The model under review builds one solid part; all positions refer to its coordinate system, in mm. A direction names the side the tool comes from. Coordinates: 2 decimals unless noted, no trailing zeros. Write each loop counter-clockwise with the first axis right and the second up, starting at its lowest first coordinate (ties: lowest second). Pieces come first, ordered by that corner, then holes. Notation, with made-up numbers: M 19.5,-17.75 L 28.5,-17.75 A37 cw 28.5,19.25 Z; hole C 58,70 d3. An arc over 180 degrees is marked long. Answer as a JSON object with one key per item and string values.
```python
from build123d import *
from build123d import SkipClean  # not in build123d's __all__

# Parameters (mm, degrees)
F1_DEPTH  = 24.13
F2_R      = 2.032
F2_R_2    = 1.2065
F3_DEPTH  = 0.7874
F4_DEPTH  = 25.4
F6_DEPTH  = 0.5
F7_DEPTH  = 2
F8_DEPTH  = 2
F9_W      = 25.654
F9_H      = 1
F10_DEPTH = 1.27
F11_R     = 1.2065
F12_DEPTH = 1.905
F13_DEPTH = 1.905
F14_DEPTH = 1.0414


# Not quite as in the source:
# - after a boolean that leaves OpenCascade's solid faulty, fix() repairs it
# - a feature names something its author has since deleted; it is built from what else it names


with BuildPart() as f1:
    # F0 (on Top) → F1 (new body)
    with BuildSketch(Plane.XY):
        Polygon((-22.881621525, -1.6067087497), (-22.881621525, 2.0254912503), (-24.151621525, 2.0254912503), (-24.151621525, -2.8767087497), (4.042378475, -2.8767087497), (4.042378475, 2.0254912503), (2.772378475, 2.0254912503), (2.772378475, -1.6067087497), align=None)
    extrude(amount=F1_DEPTH)

    # F2 (on face) → F3 (cut)
    with BuildSketch(Plane.XZ.offset(2.8767087497)):
        with Locations((-19.935221525, 12.065)):
            Circle(F2_R)
        with Locations((-19.935221525, 12.065)):
            Circle(F2_R_2, mode=Mode.SUBTRACT)
        with Locations((-0.174021525, 12.065)):
            Circle(F2_R)
        with Locations((-0.174021525, 12.065)):
            Circle(F2_R_2, mode=Mode.SUBTRACT)
    extrude(amount=-F3_DEPTH, mode=Mode.SUBTRACT)

    # F4 (cut): faces of the model
    f4_faces = [f1.faces().sort_by_distance(p)[0] for p in [
        (-19.935221525, -2.8767087497, 12.065),
        (-0.174021525, -2.8767087497, 12.065),
    ]]
    extrude(f4_faces, amount=-F4_DEPTH, mode=Mode.SUBTRACT)

    # F5 (on face) → F6 (cut)
    with BuildSketch(Plane.XZ.offset(2.8767087497)):
        Polygon((-12.3912415756, 17.8113617003), (-13.6065593278, 15.684556216), (-13.3501001609, 15.5277705701), (-14.9427792273, 12.7550959473), (-15.21558023, 12.9117982314), (-16.4524054843, 10.7586249602), (-16.6849697297, 10.6241926551), (-14.3470017528, 6.5795714036), (-14.0742704561, 6.7396221901), (-11.6537952153, 6.7396221901), (-11.6537952153, 7.0368205197), (-8.471750264, 7.0368205197), (-8.471750264, 6.7396221901), (-6.0077723583, 6.7396221901), (-5.7620638571, 6.5984823741), (-3.4414858846, 10.6383468956), (-3.6771140247, 10.7619399543), (-4.9225916905, 12.9113931759), (-5.1792576933, 12.7626708074), (-6.7848130465, 15.533548376), (-6.5128039159, 15.6911611557), (-7.7413314311, 17.8113617003), (-7.7413314311, 17.9749652743), (-12.3912415756, 17.9749652743), align=None)
        Polygon((-12.1788967651, 14.8354667667), (-11.7852579159, 15.4973436147), (-8.3281154101, 15.4973436147), (-7.9414616069, 14.830054039), (-7.6521674377, 14.9976824493), (-6.0583813106, 12.2471162856), (-6.3580625964, 12.0734691718), (-5.9656283895, 11.396203739), (-7.6865507823, 8.4002719491), (-8.471750264, 8.4002719491), (-8.471750264, 8.0795111135), (-11.6385354949, 8.0795111135), (-11.6385354949, 8.3887251094), (-12.4105562744, 8.3887251094), (-14.1476861274, 11.3866747806), (-13.7563398992, 12.0679644255), (-14.0430930461, 12.2326810967), (-12.4564279131, 14.9948861397), align=None, mode=Mode.SUBTRACT)
    extrude(amount=-F6_DEPTH, mode=Mode.SUBTRACT)

    # F7 (add): a face of the model
    f7_faces = [f1.faces().sort_by_distance(p)[0] for p in [
        (-10.054621525, -1.7395492941, 0),
    ]]
    extrude(f7_faces, amount=F7_DEPTH)

    # F8 (add): a face of the model
    f8_faces = [f1.faces().sort_by_distance(p)[0] for p in [
        (-10.054621525, -1.7395492941, 24.13),
    ]]
    extrude(f8_faces, amount=F8_DEPTH)

    # F9 (on face) → F10 (join)
    with BuildSketch(Plane(origin=(0, -1.6067087497, 0), x_dir=(-1, 0, 0), z_dir=(0, 1, 0))):
        with Locations((10.054621525, 25.63)):
            Rectangle(F9_W, F9_H)
        with Locations((10.054621525, -1.5)):
            Rectangle(F9_W, F9_H)
    extrude(amount=F10_DEPTH)

    # F11 (on face) → F12 (join)
    with BuildSketch(Plane(origin=(0, -1.6067087497, 0), x_dir=(-1, 0, 0), z_dir=(0, 1, 0))):
        with BuildLine():
            ThreePointArc((-2.772378475, 6.4958446701), (-1.4028429606, 8.7376625106), (0.8266095876, 10.1272365784))
            ThreePointArc((0.8266095876, 10.1272365784), (2.218721566, 12.065), (0.8266095876, 14.0027634216))
            ThreePointArc((0.8266095876, 14.0027634216), (-1.4028429606, 15.3923374894), (-2.772378475, 17.6341553299))
            Line((-2.772378475, 17.6341553299), (-2.772378475, 6.4958446701))
        make_face()
        with Locations((0.174021525, 12.065)):
            Circle(F11_R, mode=Mode.SUBTRACT)
        with BuildLine():
            ThreePointArc((19.2826334624, 10.1272365784), (21.5120860106, 8.7376625106), (22.881621525, 6.4958446701))
            Line((22.881621525, 6.4958446701), (22.881621525, 17.6341553299))
            ThreePointArc((22.881621525, 17.6341553299), (21.5120860106, 15.3923374894), (19.2826334624, 14.0027634216))
            ThreePointArc((19.2826334624, 14.0027634216), (17.890521484, 12.065), (19.2826334624, 10.1272365784))
        make_face()
        with Locations((19.935221525, 12.065)):
            Circle(F11_R, mode=Mode.SUBTRACT)
    with SkipClean():  # cleaning this boolean's faces spoils the solid; the shape is the same uncleaned
        extrude(amount=F12_DEPTH)

    # F13 (add): faces of the model
    f13_faces = [f1.faces().sort_by_distance(p)[0] for p in [
        (-23.516621525, 2.0254912503, 12.065),
        (-10.054621525, -0.3367087497, 25.63),
        (-10.054621525, -0.3367087497, -1.5),
        (3.407378475, 2.0254912503, 12.065),
    ]]
    extrude(f13_faces, amount=F13_DEPTH)

    add(f1.part.fix(), mode=Mode.REPLACE)

    # F14 (cut): a face of the model
    f14_faces = [f1.faces().sort_by_distance(p)[0] for p in [
        (-10.054621525, 1.5682912503, 25.63),
    ]]
    extrude(f14_faces, amount=-F14_DEPTH, mode=Mode.SUBTRACT)


solid = f1.part
```
(1) For pin 1 Ø1.5 at (x, z) = (-20, 13) entering from +Y; pin 2 Ø3 at (x, z) = (-6.5, 6) entering from +Y, all flat-tipped, find the tip position at first contact; note any pin that passes through.
Results list:
{"pin 1": "y = 0.3", "pin 2": "y = -1.61"}
(2) Add section B-B on x = -10.75. Give the boundary of the cut face in (y, z), and give its area (3 significant figures).
Results list:
{"outline": "M -2.88,-2 L 1.57,-2 L 1.57,-1 L -1.61,-1 L -1.61,25.13 L 0.53,25.13 L 0.53,26.13 L -2.88,26.13 L -2.88,17.97 L -2.38,17.97 L -2.38,15.5 L -2.88,15.5 L -2.88,8.08 L -2.38,8.08 L -2.38,7.04 L -2.88,7.04 Z", "area": "39.3 mm²"}
(3) For faces 4 (the face through (-9.9, 1.568, -1.5)), 5 (the face through (-12.99, -2.63, 16.76)), 6 (the face through (-2.22, -0.67, 12.03)), list the 3-axis set-ups (+Z, -Z, +X, -X, +Y, -Y) from which the entire face can be reached by the end or side of a thin tool; tool diameter is ignored.
Results list:
{"face 4": "+Z, -Z, +Y", "face 5": "-Y", "face 6": "+Y"}
(4) Add section C-C on z = 20. Give the boundary of the cut face in (x, y).
Results list:
{"outline": "M -24.15,-2.88 L 4.04,-2.88 L 4.04,3.93 L 2.77,3.93 L 2.77,-1.61 L -22.88,-1.61 L -22.88,3.93 L -24.15,3.93 Z"}
(5) Wall thickness on line 1 along X through (y, z) = (3, 2.5); line 2 along Z through (x, y) = (-22.25, -1.5); line 3 along Z through (x, y) = (-13, -2.5): over which ranges is each line inside the solid? List them lowest first. Write a range as from..to.
Results list:
{"line 1": "-24.15..-22.88, 2.77..4.04", "line 2": "-2..-1, 7.82..16.31, 25.13..26.13", "line 3": "-2..6.74, 9.41..14.05, 16.75..26.13"}
(6) Draft analysis for pull direction X (two halves, no side actions). For faces 1 (the face through (-21.5, 0.298, 12.1)), 2 (the face through (4.042, 0, 12)), 3 (the face through (-10, -2.877, 12)), state which applies: released by +X, released by -X, zero draft, split by the parting line, or undercut.
Results list:
{"face 1": "undercut", "face 2": "released by +X", "face 3": "zero draft"}
(7) Add section D-D on x = -21.5. Give the boundary of the cut face in (y, z), and give its area (3 significant figures).
Results list:
{"outline": "M -2.88,-2 L 1.57,-2 L 1.57,-1 L -1.61,-1 L -1.61,8.75 L 0.3,8.75 L 0.3,15.38 L -1.61,15.38 L -1.61,25.13 L 0.53,25.13 L 0.53,26.13 L -2.88,26.13 L -2.88,13.36 L -2.09,13.36 L -2.09,10.77 L -2.88,10.77 Z", "area": "51.6 mm²"}
(8) Add section A-A on y = 3. Give the boundary of the cut face in (x, z), and give its area (4 significant figures).
Results list:
{"outline": "M -24.15,-2 L -22.88,-2 L -22.88,26.13 L -24.15,26.13 Z; M 2.77,-2 L 4.04,-2 L 4.04,26.13 L 2.77,26.13 Z", "area": "71.45 mm²"}
